Autodesk Inventor part; units mm, degrees
ref_plane "YZ Plane" through (0, 0, 0) normal (1, 0, 0) x (0, 1, 0)
ref_plane "XZ Plane" through (0, 0, 0) normal (0, 1, 0) x (-1, 0, 0)
ref_plane "XY Plane" through (0, 0, 0) normal (0, 0, 1) x (1, 0, 0)
sketch "Sketch1" plane through (0, 0, 0) normal (0, 0, 1) x (1, 0, 0)
  line L0 (2.55, 4.8) -> (3.525, 5.5)
  line L1 (3.525, 5.5) -> (4.5, 4.8)
  line L2 (4.5, 4.8) -> (5, 4.8)
  line L3 (5, 4.8) -> (5, 0)
  line L4 (5, 0) -> (2.55, 0)
  line L5 (2.55, 0) -> (2.55, 4.8)
  line L6 (0, 0) -> (0, 15.358) construction
  line L7 (2.55, 4.8) -> (4.5, 4.8) construction
  point P0 (3.775, 0)
  dimension "d0" = 2.55
  dimension "d1" = 5
  dimension "d2" = 5.5
  dimension "d4" = 4.8
  dimension "d5" = 0.5
revolve "Revolution1" add sketch "Sketch1" angle 360 about axis through (0, 0, 0) along (0, 1, 0)
fillet "Fillet1" radius 0.5 2 edges at (-5, 4.8, 0) (-5, 0, 0)
sketch "Sketch2" plane through (0, 0, 0) normal (1, 0, 0) x (0, 1, 0)
  circle A0 centre (2.4833, 0) radius 1.5
  point P0 (0, 0)
  dimension "d8" = 3
extrude "Extrusion1" cut sketch "Sketch2" against normal blind 10
thread "Thread1"
properties part number "5mm Collar"
The listing builds one solid part. Answer for the finished solid, in the listing's coordinates (mm). A direction names the side the tool comes from. Round coordinates to 2 decimals unless told otherwise and drop trailing zeros. Order: outer loops, then holes, each group sorted by start corner. A loop starts at its lowest first (then second) coordinate and runs counter-clockwise, first axis right, second up. Notation, with made-up numbers: (-18, 73) - (-11, 73) arc R17 cw to (-11, 98) - close; hole circle Ø1 at (25.25, -7.75). An arc over 180 degrees is marked (long way). Write item = value, one per line. Start each with the question number.
1) For a pull along X with two mould halves and no side action, classify faces 3 (the cylindrical face through (2.43, 2.43, -0.77)), 4 (the cylindrical face through (4.77, 2.37, 1.5)), 5 (the flat face through (2, 0, 2)) as released by +X, released by -X, zero draft, split by the parting line, or undercut.
2) Given pin 1 (1.5 mm diameter, centred on x = -0.5, y = 1, fed in from +Z); pin 2 (4 mm diameter, centred on x = 0, z = 0, fed in from +Y); pin 3 (1 mm diameter, centred on x = 2.5, y = 1, fed in from -Z); pin 4 (2 mm diameter, centred on y = 2.5, z = 2, fed in from -X), each flat-ended and moving along its own axis, determine where each tip first touches the part or whether it passes through.
3) Section C-C, the plane y = 3.5 is taken. Write down the section's boundary in (x, z), plus the area to 3 significant figures.
4) Section D-D, the plane y = 1.65 is taken. Write down the section's boundary in (x, z), plus the area to 3 significant figures.
5) Straight lines are drawn through the part: L1, parallel to X at y = 3.3, z = -2; L2, parallel to Z at x = -0.75, y = 4.05; L3, parallel to X at y = 2.35, z = 0. For each, find the intervals that lie inside material, in ascending order.
6) For faces 1 (the cylindrical face through (-3.51, 3.87, -0.57)), 2 (the conical face through (-2, 5, -2)), determine the directions among +Z, -Z, +X, -X, +Y, -Y from which every point of the face is accessible in a straight line to the end or side of a thin tool.
7) Section B-B, the plane z = 0 is taken. Count the separate pieces of the cut face and the enclosed holes in it, plus the area to 3 significant figures.
Results list:
q1.face_3 = undercut
q1.face_4 = split by the parting line
q1.face_5 = zero draft
q2.pin_1 = 5
q2.pin_2 = through
q2.pin_3 = -4.58
q2.pin_4 = -4.83
q3.outline = (-4.88, -1.1) arc R5 ccw (long way) to (-4.88, 1.1) - (-2.3, 1.1) arc R2.55 cw (long way) to (-2.3, -1.1) - close
q3.area = 52.6 mm^2
q4.outline = (-4.84, -1.25) arc R5 ccw (long way) to (-4.84, 1.25) - (-2.22, 1.25) arc R2.55 cw (long way) to (-2.22, -1.25) - close
q4.area = 51.9 mm^2
q5.L1 = -4.58 to -1.58, 1.58 to 4.58
q5.L2 = -4.94 to -2.44, 2.44 to 4.94
q5.L3 = 2.55 to 5
q6.face_1 = -X
q6.face_2 = +Y
q7.separate_pieces = 3
q7.enclosed_holes = 0
q7.area = 17.3 mm^2
